Design review of the part built by this model. Coordinates are the model's own, in mm. Face numbers are marked on the shaded views. Coordinates: 2 decimals unless noted, no trailing zeros. Write item = value, one per line. Start each with the question number.
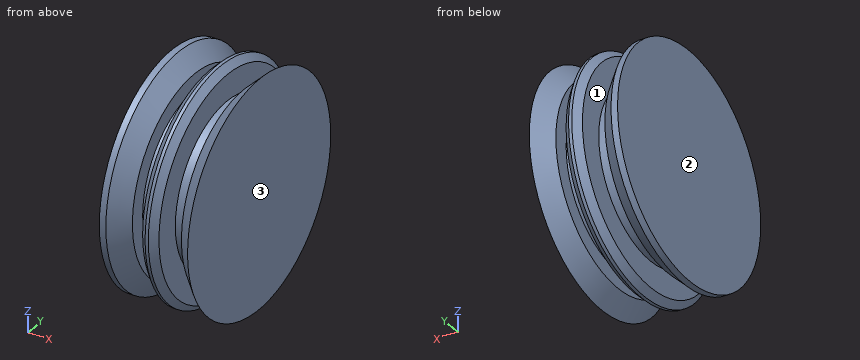
```python
from build123d import *

# Parameters (mm, degrees)
F0_R      = 35
F1_DEPTH  = 7
F2_R      = 25
F3_DEPTH  = 5
F5_R      = 35
F6_DEPTH  = 5
F7_R      = 25
F8_DEPTH  = 5
F9_R      = 35
F10_DEPTH = 5
F11_SIZE  = 4.99999
F12_SIZE  = 2


# Not quite as in the source:
# - a fillet or chamfer is up to 0.001 mm smaller than in the source, because OpenCascade refuses the exact size


with BuildPart() as f1:
    # F0 (on Right) → F1 (new body)
    with BuildSketch(Plane.YZ):
        Circle(F0_R)
    extrude(amount=F1_DEPTH)

    # F2 (on face) → F3 (join)
    with BuildSketch(Plane.YZ.offset(7)):
        Circle(F2_R)
    extrude(amount=F3_DEPTH)

    # F5 (on face) → F6 (join)
    with BuildSketch(Plane.YZ.offset(12)):
        Circle(F5_R)
    extrude(amount=F6_DEPTH)

    # F7 (on face) → F8 (join)
    with BuildSketch(Plane.YZ.offset(17)):
        Circle(F7_R)
    extrude(amount=F8_DEPTH)

    # F9 (on face) → F10 (join)
    with BuildSketch(Plane.YZ.offset(22)):
        Circle(F9_R)
    extrude(amount=F10_DEPTH)

    # F11 (size 5 in the source; OpenCascade refuses exactly that, so slightly less here)
    f11_edges = [f1.edges().sort_by_distance(p)[0] for p in [
        (7, -35, 0),
        (22, -35, 0),
    ]]
    chamfer(f11_edges, length=F11_SIZE)

    # F12
    f12_edges = [f1.edges().sort_by_distance(p)[0] for p in [
        (12, -35, 0),
        (17, -35, 0),
    ]]
    chamfer(f12_edges, length=F12_SIZE)


solid = f1.part
```
(1) For pin 1 Ø10 at (x, y) = (18, -27.5) entering from +Z; pin 2 Ø1.5 at (x, z) = (18.5, -12.5) entering from -Y; pin 3 Ø8 at (x, y) = (19.5, 12) entering from -Z, all flat-tipped, find the tip position at first contact; note any pin that passes through.
(2) Mouldability with a two-part tool opening along X and no side actions: class the marked faces 1, 2 and 3 as pulls with the +X half, pulls with the -X half, needs draft (parallel to the pull), parting line crosses it, or undercut.
(3) Take a section at C-C, the plane z = -26. Count the separate pieces of the cut face and the enclosed holes in it, then the cut area to 3 significant figures.
(4) For line 1 (X direction, y = -10.5, z = 23); line 2 (X direction, y = -28, z = 15.5); line 3 (Z direction, x = 18, y = 15), list the stretches that pass through material, from the lowest coordinate up.
Report:
q1.pin_1 = 25.94
q1.pin_2 = -22.07
q1.pin_3 = -32.57
q2.face_1 = undercut
q2.face_2 = pulls with the -X half
q2.face_3 = pulls with the +X half
q3.separate_pieces = 3
q3.enclosed_holes = 0
q3.area = 704 mm2
q4.line_1 = 0 to 7, 12 to 17, 22 to 27
q4.line_2 = 0 to 5, 12 to 17, 24 to 27
q4.line_3 = -20 to 20
